The listing builds one solid part. Answer for the finished solid, in the listing's coordinates (mm). Face numbers are marked on the shaded views. A direction names the side the tool comes from. Give positions to 0.01 mm unless a question says otherwise; leave off trailing zeros. Order: outer loops, then holes, each group sorted by start corner. A loop starts at its lowest first (then second) coordinate and runs counter-clockwise, first axis right, second up. Notation, with made-up numbers: (73.5, 53.25) -> (132.5, 53.25) arc R18 cw to (132.5, 70.25) -> close; hole circle Ø10 at (72.5, 84.25). An arc over 180 degrees is marked (long way). Write item = value, one per line. Start each with the question number.
```python
from build123d import *

# Parameters (mm, degrees)
SKETCH1_W           = 16.2306
SKETCH1_H           = 3.048
SKETCH1_R           = 1.016
BOSS_EXTRUDE1_DEPTH = 3.048


with BuildPart() as part:
    # Sketch1 → Boss-Extrude1 (new body)
    with BuildSketch(Plane(origin=(0, 0, 0), x_dir=(1, 0, 0), z_dir=(0, 1, 0))):
        Polygon((0, 8.5217), (0, -8.5217), (5.08, -8.5217), (5.08, -14.6177), (27.4066, -14.6177), (27.4066, -8.5217), (32.4866, -8.5217), (32.4866, 8.5217), (27.4066, 8.5217), (27.4066, 14.6177), (5.08, 14.6177), (5.08, 8.5217), align=None)
        with Locations((16.2433, -10.0457)):
            Rectangle(SKETCH1_W, SKETCH1_H, mode=Mode.SUBTRACT)
        with Locations((16.2433, 10.0457)):
            Rectangle(SKETCH1_W, SKETCH1_H, mode=Mode.SUBTRACT)
        with BuildLine():
            Line((30.06725, -5.9817), (2.41935, -5.9817))
            Line((2.41935, -5.9817), (2.41935, -2.54))
            ThreePointArc((2.41935, -2.54), (4.95935, 0), (2.41935, 2.54))
            Line((2.41935, 2.54), (2.41935, 5.9817))
            Line((2.41935, 5.9817), (30.06725, 5.9817))
            Line((30.06725, 5.9817), (30.06725, 2.54))
            ThreePointArc((30.06725, 2.54), (27.52725, 0), (30.06725, -2.54))
            Line((30.06725, -2.54), (30.06725, -5.9817))
        make_face(mode=Mode.SUBTRACT)
        with Locations(Location((2.41935, 0, 0), (0, 0, 90))):
            Circle(SKETCH1_R, mode=Mode.SUBTRACT)
        with Locations(Location((30.06725, 0, 0), (0, 0, 90))):
            Circle(SKETCH1_R, mode=Mode.SUBTRACT)
    extrude(amount=BOSS_EXTRUDE1_DEPTH)


solid = part.part
```
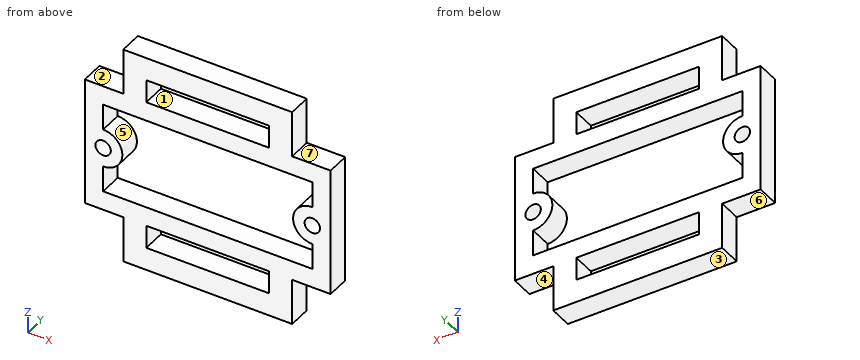
Item 1: Which of the six approach directions +Z, -Z, +X, -X, +Y, -Y give full straight-line access (tool end or side, diameter ignored) to the marked faces 3, 4, 5, 6 and 7?
Item 2: A cutting plane is placed at A-A, the plane x = 24. Write down the section's boundary in (y, z), plus the area to 3 significant figures.
Item 3: The mould has two halves that part along X. Classify the marked faces 1 and 2: +X half, -X half, draft (parallel to the pull), parting line (faces both ways), or undercut.
Item 4: A cutting plane is placed at C-C, the plane z = 0. Write down the section's boundary in (x, y), plus the area to 3 significant figures.
Item 5: A cutting plane is placed at D-D, the plane z = -5.25. Write down the section's boundary in (x, y), plus the area to 3 significant figures.
Item 6: Consider L1, parallel to Z at x = 22, y = 2.45; L2, parallel to X at y = 1.8, z = 0; L3, parallel to Z at x = 25, y = 2.05. Determine where each line is inside the solid, lowest interval first. Write a range as from..to.
Item 7: Flat-ended cylindrical pins translate along their axes: pin 1 (0.9 mm diameter, centred on y = 2, z = -10.5, fed in from +X); pin 2 (0.9 mm diameter, centred on y = 1.5, z = 9.5, fed in from -X); pin 3 (1.6 mm diameter, centred on x = 30.07, z = 0, fed in from +Y); pin 4 (0.9 mm diameter, centred on x = 30, y = 2, fed in from -Z). Find the tip coordinate at first contact, or state that the pin passes through.
Item 8: A cutting plane is placed at B-B, the plane y = 2. Count the separate pieces of the cut face and the enclosed holes in it, plus the area to 3 significant figures.
Check values:
q1.face_3 = -Z, +X, -X, +Y, -Y
q1.face_4 = -Z, +X, +Y, -Y
q1.face_5 = +Y, -Y
q1.face_6 = -Z, -X, +Y, -Y
q1.face_7 = +Z, +X, +Y, -Y
q2.outline = (0, -14.62) -> (3.05, -14.62) -> (3.05, -11.57) -> (0, -11.57) -> close; (0, -8.52) -> (3.05, -8.52) -> (3.05, -5.98) -> (0, -5.98) -> close; (0, 5.98) -> (3.05, 5.98) -> (3.05, 8.52) -> (0, 8.52) -> close; (0, 11.57) -> (3.05, 11.57) -> (3.05, 14.62) -> (0, 14.62) -> close
q2.area = 34.1 mm^2
q3.face_1 = undercut
q3.face_2 = draft
q4.outline = (0, 0) -> (1.4, 0) -> (1.4, 3.05) -> (0, 3.05) -> close; (3.44, 0) -> (4.96, 0) -> (4.96, 3.05) -> (3.44, 3.05) -> close; (27.53, 0) -> (29.05, 0) -> (29.05, 3.05) -> (27.53, 3.05) -> close; (31.08, 0) -> (32.49, 0) -> (32.49, 3.05) -> (31.08, 3.05) -> close
q4.area = 17.8 mm^2
q5.outline = (0, 0) -> (2.42, 0) -> (2.42, 3.05) -> (0, 3.05) -> close; (30.07, 0) -> (32.49, 0) -> (32.49, 3.05) -> (30.07, 3.05) -> close
q5.area = 14.7 mm^2
q6.L1 = -14.62..-11.57, -8.52..-5.98, 5.98..8.52, 11.57..14.62
q6.L2 = 0..1.4, 3.44..4.96, 27.53..29.05, 31.08..32.49
q6.L3 = -14.62..-5.98, 5.98..14.62
q7.pin_1 = 27.41
q7.pin_2 = 5.08
q7.pin_3 = through
q7.pin_4 = -8.52
q8.separate_pieces = 1
q8.enclosed_holes = 5
q8.area = 410 mm^2
